Source: CAD feature listing. Evaluate the final solid. Frame: model axes, mm. A direction names the side the tool comes from. Round coordinates to 2 decimals unless told otherwise and drop trailing zeros. Write each loop counter-clockwise with the first axis right and the second up, starting at its lowest first coordinate (ties: lowest second). Pieces come first, ordered by that corner, then holes. Notation, with made-up numbers: (7.25, -0.75) - (52.25, -0.75) arc R29 cw to (52.25, 31.25) - close; hole circle Ø11 at (66, -25). An arc over 180 degrees is marked (long way). Write item = value, one per line. Start each with the question number.
```python
from build123d import *
from build123d.topology import SkipClean

# Parameters (mm, degrees)
SKETCH_1_W               = 34
SKETCH_1_H               = 22
EXTRUDE_1_DEPTH          = 1
SKETCH_3_R               = 9
SKETCH_3_R_2             = 6
EXTRUDE_3_DEPTH          = 4
SKETCH_4_R               = 7.99
SKETCH_4_R_2             = 6
EXTRUDE_4_DEPTH          = 4
EXTRUDE_5_DEPTH          = 3
CUT_EXTRUDE_START        = -3
SKETCH_6_R               = 6
CUT_EXTRUDE_1_DEPTH      = 3
MIRROR_START             = -14
MIRROR_9_OUTLINE_R       = 6
MIRROR_9_DEPTH           = 3
EXTRUDE_START            = 1
SKETCH_7_R               = 9
SKETCH_7_R_2             = 6
EXTRUDE_6_DEPTH          = 1
EXTRUDE_START_2          = 1.9
SKETCH_8_R               = 7.99
EXTRUDE_7_DEPTH          = 1.9
EXTRUDE_START_3          = -5.9
SKETCH_9_R               = 6
EXTRUDE_8_DEPTH          = 5.9
SKETCH_10_R              = 3
CUT_EXTRUDE_2_DEPTH      = 10
CUT_EXTRUDE_3_REACH      = 47.167
SKETCH_11_R              = 1.15
PATTERN_CIRCULAR_1_COUNT = 4
SKETCH_12_R              = 2
CUT_EXTRUDE_4_DEPTH      = 2.5
PATTERN_CIRCULAR_2_COUNT = 4
CUT_EXTRUDE_5_DEPTH      = 41.635575547
CHAMFER_1_SIZE           = 1.5
SKETCH_15_W              = 8
SKETCH_15_H              = 2
CUT_EXTRUDE_8_DEPTH      = 10
EXTRUDE_9_DEPTH          = 3
SKETCH_17_W              = 8.5
SKETCH_17_H              = 21.138622828
CUT_EXTRUDE_9_DEPTH      = 1
SKETCH_18_W              = 10.48
SKETCH_18_H              = 7
SKETCH_18_W_2            = 10.5
SKETCH_18_H_2            = 6
CUT_EXTRUDE_10_DEPTH     = 33.714675606
CHAMFER_2_SIZE           = 2
SKETCH_19_R              = 3
CUT_EXTRUDE_11_DEPTH     = 33.714675606
SKETCH_20_R              = 1.15
CUT_EXTRUDE_12_DEPTH     = 33.714675606
SKETCH_23_W              = 1.26
SKETCH_23_H              = 2
SKETCH_23_H_2            = 2.235993873
EXTRUDE_10_DEPTH         = 3
CUT_EXTRUDE_14_DEPTH     = 43.898135158
CHAMFER_3_SIZE           = 1


# Read off the part's stored shape, not the designer's step: the mirror step
with BuildPart() as part:
    # Sketch 1 → Extrude 1 (new, symmetric)
    with BuildSketch(Plane.XY):
        Rectangle(SKETCH_1_W, SKETCH_1_H)
    extrude(amount=EXTRUDE_1_DEPTH, both=True)



with BuildPart() as body_2:
    # Sketch 3 → Extrude 3 (new body)
    with BuildSketch(Plane(origin=(0, 11, 0), x_dir=(1, 0, 0), z_dir=(0, 1, 0))):
        with Locations(Location((-7.5, 12.5, 0), (0, 0, 180))):
            Circle(SKETCH_3_R)
        with Locations(Location((-7.5, 12.5, 0), (0, 0, 180))):
            Circle(SKETCH_3_R_2, mode=Mode.SUBTRACT)
    extrude(amount=EXTRUDE_3_DEPTH)

    # Sketch 4 → Extrude 4 (add)
    with BuildSketch(Plane(origin=(0, 15, 0), x_dir=(1, 0, 0), z_dir=(0, 1, 0))):
        with Locations(Location((-7.5, 12.5, 0), (0, 0, 180))):
            Circle(SKETCH_4_R)
        with Locations(Location((-7.5, 12.5, 0), (0, 0, 180))):
            Circle(SKETCH_4_R_2, mode=Mode.SUBTRACT)
    extrude(amount=EXTRUDE_4_DEPTH)


with BuildPart() as part_1:
    add(part.part)

    add(body_2.part)  # Extrude 5 merges body 2
    # Sketch 5 → Extrude 5 (add)
    with BuildSketch(Plane(origin=(0, 11, 0), x_dir=(1, 0, 0), z_dir=(0, 1, 0))):
        with BuildLine():
            Line((17, -1), (17, 5))
            Line((17, 5), (-2.010591436, 19.632067976))
            ThreePointArc((-2.010591436, 19.632067976), (-11.47462721, 20.574796501), (-16.5, 12.5))
            Line((-16.5, 12.5), (-17, 1))
            Line((-17, 1), (-17, -1))
            Line((-17, -1), (17, -1))
        make_face()
    extrude(amount=EXTRUDE_5_DEPTH)

    # Sketch 6 → Cut-Extrude 1 (cut)
    with BuildSketch(Plane(origin=(0, 14, 0), x_dir=(1, 0, 0), z_dir=(0, 1, 0)).offset(CUT_EXTRUDE_START)):
        with Locations(Location((-7.5, 12.5, 0), (0, 0, 180))):
            Circle(SKETCH_6_R)
    extrude(amount=CUT_EXTRUDE_1_DEPTH, mode=Mode.SUBTRACT)

    # Mirror 9 outline → Mirror 9 (add)
    with BuildSketch(Plane(origin=(0, 0, 0), x_dir=(1, 0, 0), z_dir=(0, 1, 0)).offset(MIRROR_START)):
        with BuildLine():
            Line((-17, 1), (-17, -1))
            Line((-17, -1), (17, -1))
            Line((17, -1), (17, 5))
            Line((17, 5), (-2.010591436, 19.632067976))
            ThreePointArc((-2.010591436, 19.632067976), (-11.47462721, 20.574796501), (-16.5, 12.5))
            Line((-16.5, 12.5), (-17, 1))
        make_face()
        with Locations((-7.5, 12.5)):
            Circle(MIRROR_9_OUTLINE_R, mode=Mode.SUBTRACT)
    extrude(amount=MIRROR_9_DEPTH)

    # Sketch 7 → Extrude 6 (add)
    with SkipClean():  # the faces are left unmerged after this step: merging them gives an invalid solid
        with BuildSketch(Plane.XZ.offset(14).offset(EXTRUDE_START)):
            with Locations(Location((-7.5, -12.5, 0), (0, 0, 180))):
                Circle(SKETCH_7_R)
            with Locations(Location((-7.5, -12.5, 0), (0, 0, 180))):
                Circle(SKETCH_7_R_2, mode=Mode.SUBTRACT)
        extrude(amount=-EXTRUDE_6_DEPTH)

    # Sketch 8 → Extrude 7 (add)
    with SkipClean():  # the faces are left unmerged after this step: merging them gives an invalid solid
        with BuildSketch(Plane.XZ.offset(15).offset(EXTRUDE_START_2)):
            with Locations(Location((-7.5, -12.5, 0), (0, 0, 180))):
                Circle(SKETCH_8_R)
        extrude(amount=-EXTRUDE_7_DEPTH)

    # Sketch 9 → Extrude 8 (add)
    with BuildSketch(Plane(origin=(0, -11, 0), x_dir=(1, 0, 0), z_dir=(0, 1, 0)).offset(EXTRUDE_START_3)):
        with Locations(Location((-7.5, 12.5, 0), (0, 0, 180))):
            Circle(SKETCH_9_R)
    extrude(amount=EXTRUDE_8_DEPTH)

    # Sketch 10 → Cut-Extrude 2 (cut)
    with BuildSketch(Plane.XZ.offset(16.9)):
        with Locations((-7.5, -12.5)):
            Circle(SKETCH_10_R)
    extrude(amount=-CUT_EXTRUDE_2_DEPTH, mode=Mode.SUBTRACT)

    # Sketch 11 → Cut-Extrude 3 (cut, up to next)
    with BuildSketch(Plane.XZ.offset(16.9), mode=Mode.PRIVATE) as cut_extrude_3_sk1:
        with Locations((-7.5, -18.5)):
            Circle(SKETCH_11_R)
    cut_extrude_3_tool1 = extrude(cut_extrude_3_sk1.sketch, amount=-CUT_EXTRUDE_3_REACH, mode=Mode.PRIVATE) & part_1.part
    cut_extrude_3 = cut_extrude_3_tool1.solids().sort_by_distance((-7.5, -16.9, -18.5))[0]
    add(cut_extrude_3, mode=Mode.SUBTRACT)

    # Pattern Circular 1: Cut-Extrude 3 ×4 about axis
    pattern_circular_1_axis = Axis((-7.5, 0, -12.5), (0, 1, 0))
    for i in range(1, PATTERN_CIRCULAR_1_COUNT):
        add(cut_extrude_3.rotate(pattern_circular_1_axis, i * 360 / PATTERN_CIRCULAR_1_COUNT), mode=Mode.SUBTRACT)

    # Sketch 12 → Cut-Extrude 4 (cut)
    with BuildSketch(Plane(origin=(0, -11, 0), x_dir=(1, 0, 0), z_dir=(0, 1, 0))):
        with Locations(Location((-7.5, 18.5, 0), (0, 0, 180))):
            Circle(SKETCH_12_R)
    cut_extrude_4 = extrude(amount=-CUT_EXTRUDE_4_DEPTH, mode=Mode.SUBTRACT)

    # Pattern Circular 2: Cut-Extrude 4 ×4 about axis
    pattern_circular_2_axis = Axis((-7.5, 0, -12.5), (0, 1, 0))
    for i in range(1, PATTERN_CIRCULAR_2_COUNT):
        add(cut_extrude_4.rotate(pattern_circular_2_axis, i * 360 / PATTERN_CIRCULAR_2_COUNT), mode=Mode.SUBTRACT)

    # Sketch 14 → Cut-Extrude 5 (cut, through all)
    with BuildSketch(Plane(origin=(0, -11, 0), x_dir=(1, 0, 0), z_dir=(0, 1, 0))):
        Polygon((17, 5), (4.75, 14.428577397), (4.75, 1), (17, 1), align=None)
    extrude(amount=-CUT_EXTRUDE_5_DEPTH, mode=Mode.SUBTRACT)

    # Chamfer 1
    chamfer_1_edges = [part_1.edges().sort_by_distance(p)[0] for p in [
        (17, 14, -2),
    ]]
    chamfer(chamfer_1_edges, length=CHAMFER_1_SIZE)

    # Sketch 15 → Cut-Extrude 8 (cut)
    with BuildSketch(Plane(origin=(0, 0, -1), x_dir=(-1, 0, 0), z_dir=(0, 0, -1))):
        with Locations((-13, -13)):
            Rectangle(SKETCH_15_W, SKETCH_15_H)
    extrude(amount=-CUT_EXTRUDE_8_DEPTH, mode=Mode.SUBTRACT)

    # Sketch 16 → Extrude 9 (add)
    with BuildSketch(Plane(origin=(0, 0, -1), x_dir=(-1, 0, 0), z_dir=(0, 0, -1))):
        Polygon((-17, -9), (-6.73, -9), (-6.73, -14), (-9, -14), (-9, -12), (-17, -12), align=None)
    extrude(amount=EXTRUDE_9_DEPTH)

    # Sketch 17 → Cut-Extrude 9 (cut)
    with BuildSketch(Plane(origin=(0, -11, 0), x_dir=(1, 0, 0), z_dir=(0, 1, 0))):
        with Locations((0.5, 11.569311414)):
            Rectangle(SKETCH_17_W, SKETCH_17_H)
    extrude(amount=-CUT_EXTRUDE_9_DEPTH, mode=Mode.SUBTRACT)

    # Sketch 18 → Cut-Extrude 10 (cut, through all)
    with BuildSketch(Plane(origin=(0, 0, -1), x_dir=(-1, 0, 0), z_dir=(0, 0, -1))):
        with Locations((-1.49, -8.5)):
            Rectangle(SKETCH_18_W, SKETCH_18_H)
        with Locations((-1.5, 8)):
            Rectangle(SKETCH_18_W_2, SKETCH_18_H_2)
    extrude(amount=-CUT_EXTRUDE_10_DEPTH, mode=Mode.SUBTRACT)

    # Chamfer 2
    chamfer_2_edges = [part_1.edges().sort_by_distance(p)[0] for p in [
        (17, -12, -1.5),
    ]]
    chamfer(chamfer_2_edges, length=CHAMFER_2_SIZE)

    # Sketch 19 → Cut-Extrude 11 (cut, through all)
    with BuildSketch(Plane(origin=(0, 0, -1), x_dir=(-1, 0, 0), z_dir=(0, 0, -1))):
        with Locations((7.5, 1)):
            Circle(SKETCH_19_R)
    extrude(amount=-CUT_EXTRUDE_11_DEPTH, mode=Mode.SUBTRACT)

    # Sketch 20 → Cut-Extrude 12 (cut, through all)
    with BuildSketch(Plane(origin=(0, 0, -1), x_dir=(-1, 0, 0), z_dir=(0, 0, -1))):
        with Locations((15, 9)):
            Circle(SKETCH_20_R)
        with Locations((-15, 9)):
            Circle(SKETCH_20_R)
        with Locations((-15, -7)):
            Circle(SKETCH_20_R)
        with Locations((15, -7)):
            Circle(SKETCH_20_R)
    extrude(amount=-CUT_EXTRUDE_12_DEPTH, mode=Mode.SUBTRACT)

    # Sketch 23 → Extrude 10 (add)
    with BuildSketch(Plane(origin=(0, 0, -1), x_dir=(-1, 0, 0), z_dir=(0, 0, -1))):
        with Locations((16.37, -10)):
            Rectangle(SKETCH_23_W, SKETCH_23_H)
        with Locations((4.38, -9.882003064)):
            Rectangle(SKETCH_23_W, SKETCH_23_H_2)
    extrude(amount=EXTRUDE_10_DEPTH)

    # Sketch 24 → Cut-Extrude 14 (cut, through all)
    with BuildSketch(Plane.XZ.offset(14)):
        Polygon((-17, -1), (-16.869565217, -4), (-17, -4), align=None)
    extrude(amount=-CUT_EXTRUDE_14_DEPTH, mode=Mode.SUBTRACT)

    # Chamfer 3
    # the kernel refuses this chamfer: 1 mm, written as the material it takes off along each edge
    with BuildSketch(Plane(origin=(-19.571682988, 14, 1), x_dir=(0, -0.9996219169112968, 0.027495876610586296), z_dir=(1, 0, 0))) as chamfer_3_piece_1:
        Polygon((CHAMFER_3_SIZE * 0.999621916911, CHAMFER_3_SIZE * 0.0274958766106), (-CHAMFER_3_SIZE * 0.0274958766106, CHAMFER_3_SIZE * 0.999621916911), (0, 0), align=None)
    extrude(amount=37.643365976, mode=Mode.SUBTRACT)
    with BuildSketch(Plane(origin=(-19.571682988, -14, 1), x_dir=(0, 0.9996219169112968, 0.027495876610586296), z_dir=(1, 0, 0))) as chamfer_3_piece_2:
        Polygon((CHAMFER_3_SIZE * 0.999621916911, -CHAMFER_3_SIZE * 0.0274958766106), (-CHAMFER_3_SIZE * 0.0274958766106, -CHAMFER_3_SIZE * 0.999621916911), (0, 0), align=None)
    extrude(amount=31.143365976, mode=Mode.SUBTRACT)
    with BuildSketch(Plane(origin=(-17, -16.571682988, 1), x_dir=(0.9996219169112968, 0, 0.027495876610586296), z_dir=(0, 1, 0))) as chamfer_3_piece_3:
        Polygon((CHAMFER_3_SIZE * 0.999621916911, CHAMFER_3_SIZE * 0.0274958766106), (-CHAMFER_3_SIZE * 0.0274958766106, CHAMFER_3_SIZE * 0.999621916911), (0, 0), align=None)
    extrude(amount=33.143365976, mode=Mode.SUBTRACT)


solid = part_1.part
```
(1) Ray query, L1, parallel to Z at x = -7.5, y = -14.15; L2, parallel to Y at x = -15, z = -0.5; L3, parallel to Z at x = -7.5, y = -12.65. Return the intervals inside material, ascending. Write a range as from..to.
(2) Pull-direction query (X, two-part tool) for faces 5 (the cylindrical face through (-9.498, -12.232, -6.588)), 6 (the flat face through (-16.5, -0.2, 0.5)), 7 (the flat face through (-4, -10, -4)); classes: +X half, -X half, draft (parallel to the pull), parting line (faces both ways), or undercut.
(3) Contact query for flat-ended pins moving along their axis: P1, Ø3.5, axis at x = -7.5, z = -12.5, coming from the +Y side; P2, Ø6, axis at y = 5, z = -1.5, coming from the -X side; P3, Ø5, axis at x = 8, z = -1.5, coming from the -Y side; P4, Ø1, axis at x = 5.5, y = -13, coming from the -Z side. Output: stop coordinate, or through.
(4) Section D-D (y = 1.5). Return the cut outline in (x, z).
(5) Section C-C (x = -11). Return the cut outline in (y, z).
(6) Section B-B (z = -2). Return the cut outline in (x, y).
(7) Section A-A (y = -7). Return the cut outline in (x, z), plus the area to 3 significant figures.
(8) Reachability of faces 1 (the flat face through (9, -13, -1)), 2 (the flat face through (-6, -13.5, -7)), 3 (the flat face through (11, -11, -4)), 4 (the flat face through (-4, -8.764, -2)) from +Z, -Z, +X, -X, +Y, -Y: full face, straight path, thin tool, end or side. Return the list, or none.
Solution:
q1.L1 = -21.5..-19.65, -17.35..-15.5, -9.5..-7.65, -5.35..-3.5
q1.L2 = -14..-8.15, -5.85..7.85, 10.15..14
q1.L3 = -21.5..-20.5, -16.5..-15.5, -9.5..-8.5, -4.5..1
q2.face_5 = undercut
q2.face_6 = -X half
q2.face_7 = draft
q3.P1 = through
q3.P2 = -17
q3.P3 = -14
q3.P4 = -1
q4.outline = (-17, -1) - (-10.46, -1) - (-10.46, 1) - (-16, 1) - (-17, 0) - close; (-4.54, -1) - (17, -1) - (17, 1) - (-4.54, 1) - close
q5.outline = (-16.9, -19.68) - (-15, -19.68) - (-15, -20.79) - (-11, -20.79) - (-11, -1) - (11, -1) - (11, -7.63) - (19, -7.63) - (19, -5.32) - (15, -5.32) - (15, -4.21) - (14, -4.21) - (14, 0) - (13, 1) - (-13, 1) - (-14, 0) - (-14, -4.21) - (-15, -4.21) - (-15, -5.32) - (-16.9, -5.32) - close; (11, -20.79) - (15, -20.79) - (15, -19.68) - (19, -19.68) - (19, -17.37) - (11, -17.37) - close
q6.outline = (-16.96, -14) - (4.75, -14) - (4.75, -12) - (-3.75, -12) - (-3.75, -8.76) - (-5.01, -8.76) - (-5.01, -11) - (-15.74, -11) - (-15.74, -9) - (-16.96, -9) - close; (-16.96, 11) - (17, 11) - (17, 12.5) - (15.5, 14) - (-16.96, 14) - close; (6.73, -14) - (9, -14) - (9, -12) - (15, -12) - (17, -10) - (17, -9) - (6.73, -9) - close
q7.outline = (-17, -1) - (-16.15, -1) - (-16.15, 0.85) - (-17, 0) - close; (-13.85, -1) - (-3.75, -1) - (-3.75, 1) - (-13.85, 1) - close; (6.73, -1) - (13.85, -1) - (13.85, 1) - (6.73, 1) - close; (16.15, -1) - (17, -1) - (17, 1) - (16.15, 1) - close
q7.area = 37.4 mm^2
q8.face_1 = +Z, -Z, +X, -Y
q8.face_2 = none
q8.face_3 = -Z, +X, -Y
q8.face_4 = -Z, +X, -X
